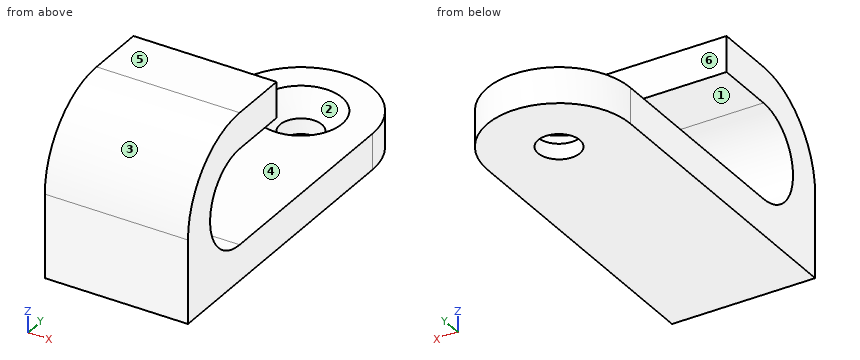
```python
from build123d import *

# Parameters (mm, degrees)
F1_DEPTH = 3
F3_DEPTH = 12
F4_SIZE  = 1.7


with BuildPart() as f1:
    # F0 (on Top) → F1 (new body)
    with BuildSketch(Plane.XY):
        with BuildLine():
            Line((6, -12.5), (6, 12.5))
            ThreePointArc((6, 12.5), (0, 6.5), (-6, 12.5))
            Line((-6, 12.5), (-6, -12.5))
            Line((-6, -12.5), (6, -12.5))
        make_face()
        with BuildLine():
            ThreePointArc((-1.75, 12.5), (0, 14.25), (1.75, 12.5))
            Line((1.75, 12.5), (6, 12.5))
            ThreePointArc((6, 12.5), (0, 18.5), (-6, 12.5))
            Line((-6, 12.5), (-1.75, 12.5))
        make_face()
        with BuildLine():
            Line((6, 12.5), (1.75, 12.5))
            ThreePointArc((1.75, 12.5), (0, 10.75), (-1.75, 12.5))
            Line((-1.75, 12.5), (-6, 12.5))
            ThreePointArc((-6, 12.5), (0, 6.5), (6, 12.5))
        make_face()
    extrude(amount=F1_DEPTH)

    # F2 (on face) → F3 (join, through all)
    with BuildSketch(Plane(origin=(-6, 0, 0), x_dir=(0, -1, 0), z_dir=(-1, 0, 0))):
        with BuildLine():
            Line((12.5, 3), (12.5, 7))
            ThreePointArc((12.5, 7), (10.4497474683, 11.9497474683), (5.5, 14))
            Line((5.5, 14), (0.5, 14))
            Line((0.5, 14), (0.5, 11))
            Line((0.5, 11), (5.5, 11))
            ThreePointArc((5.5, 11), (9.5, 7), (5.5, 3))
            Line((5.5, 3), (12.5, 3))
        make_face()
    extrude(amount=-F3_DEPTH)

    # F4
    f4_edges = [f1.edges().sort_by_distance(p)[0] for p in [
        (1.75, 12.5, 3),
    ]]
    chamfer(f4_edges, length=F4_SIZE)


solid = f1.part
```
Geometry check sheet. Reference: the model listing, model coordinates, mm. Face numbers are marked on the shaded views. A direction names the side the tool comes from. Round coordinates to 2 decimals unless told otherwise and drop trailing zeros. Loops run counter-clockwise (first coordinate to the right, second up) from the corner with the lowest first, then second, coordinate; pieces in that order, holes last. Notation, with made-up numbers: (22.5, -24) -> (68.5, -24) arc R18 cw to (68.5, 10) -> close; hole circle Ø9 at (-37, 42). An arc over 180 degrees is marked (long way). Use a Markdown table: item, result.
(1) Sectioned sample at B-B (x = 5). Enter the section's corners in (y, z), then the cut area to 3 significant figures.
Calculated:
| item | result |
|---|---|
| outline | (-12.5, 0) -> (15.82, 0) -> (15.82, 3) -> (-5.5, 3) arc R4 cw to (-5.5, 11) -> (-0.5, 11) -> (-0.5, 14) -> (-5.5, 14) arc R7 ccw to (-12.5, 7) -> close |
| area | 141 mm² |
(2) Set-up check for the marked faces 4, 5 and 6: record each of +Z, -Z, +X, -X, +Y, -Y from which the full face is reachable in a straight line by a thin tool's end or side.
Calculated:
| item | result |
|---|---|
| face 4 | +X, -X, +Y |
| face 5 | +Z, +X, -X, +Y, -Y |
| face 6 | +Z, +X, -X, +Y |
(3) Mould release check, pull along Y, two halves, no side actions. Record for the marked faces 1, 2 and 3: released by +Y, released by -Y, zero draft, split by the parting line, or undercut.
Calculated:
| item | result |
|---|---|
| face 1 | zero draft |
| face 2 | undercut |
| face 3 | released by -Y |
(4) Sectioned sample at A-A (x = 0). Enter the section's corners in (y, z).
Calculated:
| item | result |
|---|---|
| outline | (-12.5, 0) -> (10.75, 0) -> (10.75, 1.3) -> (9.05, 3) -> (-5.5, 3) arc R4 cw to (-5.5, 11) -> (-0.5, 11) -> (-0.5, 14) -> (-5.5, 14) arc R7 ccw to (-12.5, 7) -> close; (14.25, 0) -> (18.5, 0) -> (18.5, 3) -> (15.95, 3) -> (14.25, 1.3) -> close |
(5) Scan lines: probe 1 along Y at (x, z) = (0, 0.55); probe 2 along Z at (x, y) = (-1, -1); probe 3 along Z at (x, y) = (-1.75, 6). Record each from-to range of solid material in increasing order.
Calculated:
| item | result |
|---|---|
| probe 1 | -12.5 to 10.75, 14.25 to 18.5 |
| probe 2 | 0 to 3, 11 to 14 |
| probe 3 | 0 to 3 |
(6) Go/stop test with flat-tipped pins: P1, Ø2, axis at x = 3.5, z = 2.5, coming from the +Y side; P2, Ø3, axis at x = 0, y = 12.5, coming from the -Z side; P3, Ø1, axis at x = -0.5, z = 11, coming from the +Y side; P4, Ø1, axis at x = 4, z = 5.5, coming from the +Y side. Record where each tip stops, or that it passes through.
Calculated:
| item | result |
|---|---|
| P1 | y = 17.95 |
| P2 | through |
| P3 | y = -0.5 |
| P4 | y = -8.96 |
(7) Sectioned sample at D-D (z = 5.5). Enter the section's corners in (x, y).
Calculated:
| item | result |
|---|---|
| outline | (-6, -12.5) -> (6, -12.5) -> (6, -9.21) -> (-6, -9.21) -> close |
(8) Sectioned sample at C-C (y = 8.5). Enter the section's corners in (x, z).
Calculated:
| item | result |
|---|---|
| outline | (-6, 0) -> (6, 0) -> (6, 3) -> (-6, 3) -> close |
